Build history of the part. All positions in model axes, mm. Face numbers are marked on the shaded views. A direction names the side the tool comes from. Round coordinates to 2 decimals unless told otherwise and drop trailing zeros. Write each loop counter-clockwise with the first axis right and the second up, starting at its lowest first coordinate (ties: lowest second). Pieces come first, ordered by that corner, then holes.
1) Pull direction Z, two halves, no side cores. Call the marked faces 1, 2 and 3: +Z half, -Z half, draft (parallel to the pull), parting line (faces both ways), or undercut.
2) Which spindle directions (+Z, -Z, +X, -X, +Y, -Y) get a long thin tool onto all of the face, cutting with end or side? Do the marked faces 4 and 5. Say none if no direction does.
3) Flat gauge pins, fed straight in: pin 1 (2.5 mm diameter, centred on x = 2, z = 1, fed in from +Y); pin 2 (6 mm diameter, centred on y = 55, z = 9, fed in from -X); pin 3 (6 mm diameter, centred on y = 48.5, z = 5.5, fed in from +X). Where does each tip first touch, or does it go through?
4) Wall check: probe 1 along Z at (x, y) = (0, 66); probe 2 along Z at (x, y) = (1.5, 77.5). Give the ranges that are in metal, low to high.
5) Saw through at A-A (y = 80.5). Write the cut outline in (x, z).
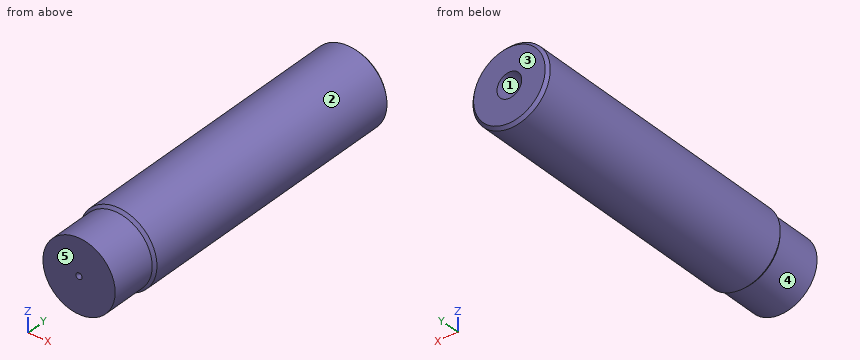
Solid Edge part; units mm, degrees
sketch "Sketch1" plane through (0, 0, 0) normal (0, 0, 1) x (1, 0, 0)
  line L0 (0, 95) -> (11.58, 95)
  line L1 (11.58, 95) -> (12.5, 94.08)
  line L2 (12.5, 94.08) -> (12.5, 0.92)
  line L3 (12.5, 0.92) -> (11.58, 0)
  line L4 (11.58, 0) -> (0, 0)
  line L5 (0, 0) -> (0, 95)
revolve "RevolvedProtrusion1" add sketch "Sketch1" angle 360 about axis through (0, 0, 0) along (0, 1, 0)
cosmetic_thread "Thread1"
sketch "Sketch2" plane through (0, 0, 0) normal (0, 0, 1) x (1, 0, 0)
  line L0 (0, 95) -> (4, 95)
  line L1 (4, 95) -> (4, 0)
  line L2 (4, 0) -> (0, 0)
  line L3 (0, 0) -> (0, 95)
revolve "RevolvedCutout1" cut sketch "Sketch2" angle 360 about axis through (0, 0, 0) along (0, 1, 0)
sketch "Sketch3" plane through (0, 0, 0) normal (0, 0, 1) x (1, 0, 0)
  line L0 (0, 0) -> (11.688, 0)
  line L1 (11.688, 0) -> (11.688, -15)
  line L2 (11.688, -15) -> (1, -15)
  line L3 (1, -15) -> (0, -14)
  line L4 (0, -14) -> (0, 0)
revolve "RevolvedProtrusion2" add sketch "Sketch3" angle 360 about axis through (0, -14, 0) along (0, 1, 0)
Evaluation:
1. face 1: undercut
1. face 2: parting line
1. face 3: draft
2. face 4: -Y
2. face 5: +Z, -Z, +X, -X, -Y
3. pin 1: stops at y = 0
3. pin 2: stops at x = -10.97
3. pin 3: stops at x = 12.25
4. probe 1: z = -12.5 to -4, 4 to 12.5
4. probe 2: z = -12.41 to -3.71, 3.71 to 12.41
5. outline: circle Ø25 at (0, 0); hole circle Ø8 at (0, 0)
